Geometry: see drawing. Coordinates: mm, zero at the bounding-box minimum. A direction names the side the tool comes from. Round coordinates to 2 decimals unless told otherwise and drop trailing zeros. Loops run counter-clockwise (first coordinate to the right, second up) from the corner with the lowest first, then second, coordinate; pieces in that order, holes last. Notation, with made-up numbers: (-19, 33) - (30, 33) arc R17 cw to (30, 65) - close; hole circle Ø8 at (53.25, 61). An arc over 180 degrees is marked (long way). Use CSV: the item, a comma, the result in double quotes.
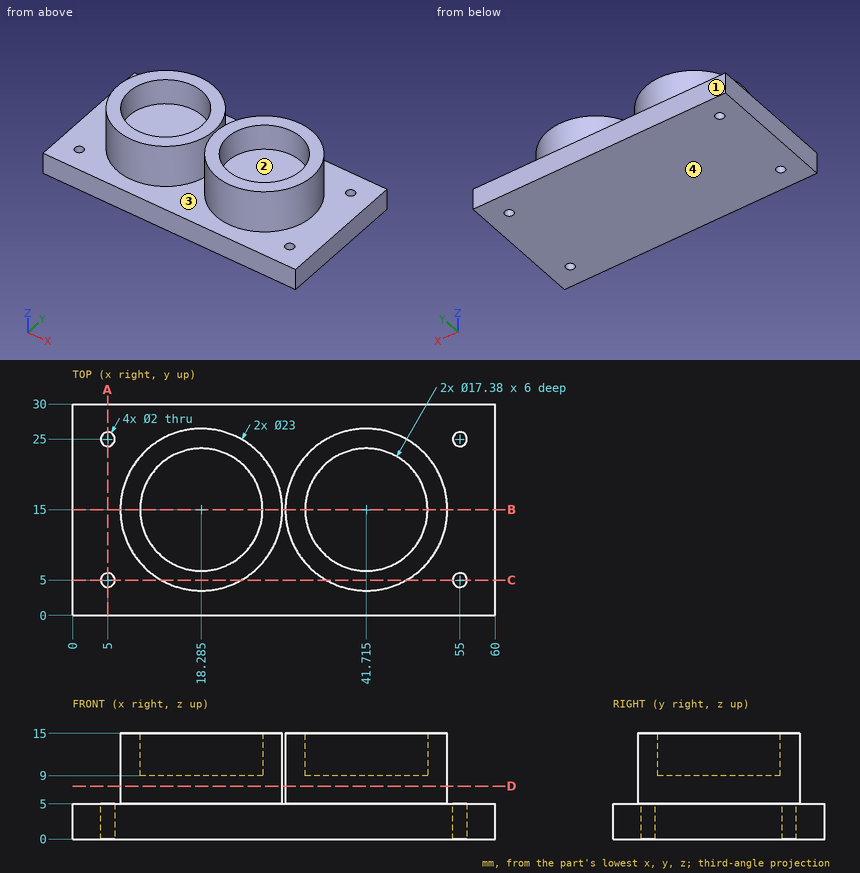
Item 1: Section C-C on y = 5. Return the cut outline in (x, z).
Final values:
outline,"(0, 0) - (4, 0) - (4, 5) - (0, 5) - close; (6, 0) - (54, 0) - (54, 5) - (47.39, 5) - (47.39, 15) - (36.04, 15) - (36.04, 5) - (23.96, 5) - (23.96, 15) - (12.61, 15) - (12.61, 5) - (6, 5) - close; (56, 0) - (60, 0) - (60, 5) - (56, 5) - close"
Item 2: Pin query (flat end, axial travel): P1, Ø5, axis at y = 22.5, z = 11.5, coming from the -X side; P2, Ø4, axis at y = 5, z = 9, coming from the -X side; P3, Ø14, axis at x = 41.715, y = 15, coming from the +Z side. Return the tip coordinate at first contact, or that it passes through.
Final values:
P1,"stops at x = 7.93"
P2,"stops at x = 10.02"
P3,"stops at z = 9"
Item 3: Section D-D on z = 7.5. Return the cut outline in (x, y) (3 decimals).
Final values:
outline,"circle Ø23 at (18.285, 15); circle Ø23 at (41.715, 15)"
Item 4: Section B-B on y = 15. Return the cut outline in (x, z) (3 decimals), plus the area to 3 significant figures.
Final values:
outline,"(0, 0) - (60, 0) - (60, 5) - (53.215, 5) - (53.215, 15) - (50.405, 15) - (50.405, 9) - (33.025, 9) - (33.025, 15) - (30.215, 15) - (30.215, 5) - (29.785, 5) - (29.785, 15) - (26.975, 15) - (26.975, 9) - (9.595, 9) - (9.595, 15) - (6.785, 15) - (6.785, 5) - (0, 5) - close"
area,"551 mm²"
Item 5: Material intervals for line 1 (Y direction, x = 55, z = 1.6); line 2 (X direction, y = 18, z = 14); line 3 (X direction, y = 14.25, z = 11.25), sorted ascending.
Final values:
line 1,"y = 0 to 4, 6 to 24, 26 to 30"
line 2,"x = 7.18 to 10.13, 26.44 to 29.39, 30.61 to 33.56, 49.87 to 52.82"
line 3,"x = 6.81 to 9.63, 26.94 to 29.76, 30.24 to 33.06, 50.37 to 53.19"
Item 6: Reachability of the marked faces 1 and 2 from +Z, -Z, +X, -X, +Y, -Y: full face, straight path, thin tool, end or side. Return the list, or none.
Final values:
face 1,"+Z, -Z, +X, -X, +Y"
face 2,"+Z"
Item 7: Section A-A on x = 5. Return the cut outline in (y, z), plus the area to 3 significant figures.
Final values:
outline,"(0, 0) - (4, 0) - (4, 5) - (0, 5) - close; (6, 0) - (24, 0) - (24, 5) - (6, 5) - close; (26, 0) - (30, 0) - (30, 5) - (26, 5) - close"
area,"130 mm²"
Item 8: Mould query, pull axis X, two halves, no side actions, for the marked faces 3 and 4. Classes: released by +X, released by -X, zero draft, split by the parting line, or undercut.
Final values:
face 3,"undercut"
face 4,"zero draft"
